Could you check a few things on this model? Use its own coordinates, in mm. Face numbers are marked on the shaded views. Coordinates: 2 decimals unless noted, no trailing zeros. Order: outer loops, then holes, each group sorted by start corner. A loop starts at its lowest first (then second) coordinate and runs counter-clockwise, first axis right, second up. Notation, with made-up numbers: (67.25, 88) -> (94.25, 88) arc R8 ccw to (94.25, 93) -> close; hole circle Ø6 at (3, 27). An arc over 180 degrees is marked (long way). Put each result on its own line as item: value. Start each with the question number.
Q1. If we section it at A-A (x = -5): Please give me the cut outline in (y, z).
Q2. If we section it at B-B (y = -1.25): Please give me the cut outline in (x, z).
Q3. We'd pull the mould along X, two halves only. Please class the marked faces 1, 2, 3 and 4: +X half, -X half, draft (parallel to the pull), parting line (faces both ways), or undercut.
Q4. Will these pins go through, and if not, where does the flat tip stop? pin 1 (1.5 mm diameter, centred on x = -0.5, y = -8.5, fed in from +Z); pin 2 (5 mm diameter, centred on x = -2.5, y = 8, fed in from -Z); pin 3 (2.5 mm diameter, centred on y = 10, z = 2.5, fed in from +X).
Q5. Please list where these lines run through material, in increasing order: line 1 along Y through (x, z) = (-15.2, 2.5); line 2 along Y through (x, z) = (0.5, 7.75); line 3 along Y through (x, z) = (15.35, 2.5).
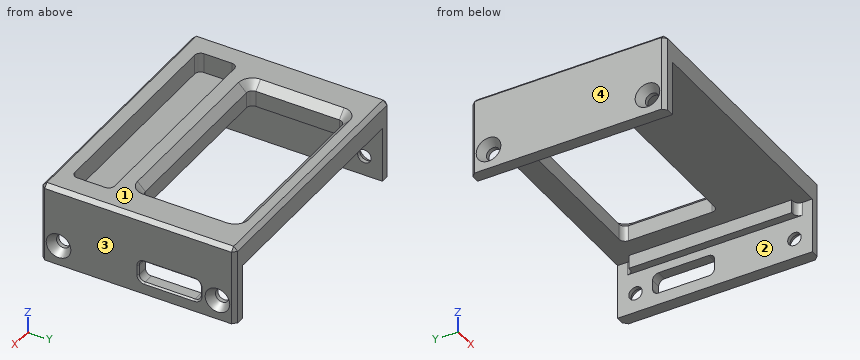
from build123d import *

# Parameters (mm, degrees)
SKETCH1_W           = 32.8
SKETCH1_H           = 24.5
BOSS_EXTRUDE1_DEPTH = 10
SKETCH3_W           = 29.8
SKETCH3_H           = 24.5
CUT_EXTRUDE2_DEPTH  = 5.3
CUT_EXTRUDE3_DEPTH  = 23.782065315
CUT_EXTRUDE4_DEPTH  = 1.5
CHAMFER1_SIZE       = 1
CHAMFER2_SIZE       = 0.2
CHAMFER3_SIZE       = 0.5
CUT_EXTRUDE6_DEPTH  = 2.5
SKETCH10_R          = 0.85
CUT_EXTRUDE7_DEPTH  = 1.5
CUT_EXTRUDE8_START  = -1.5
SKETCH9_R           = 0.85
CUT_EXTRUDE8_DEPTH  = 1.5
CHAMFER7_SIZE       = 0.7
CHAMFER7_SIZE2      = 0.999703605
CHAMFER8_SIZE       = 0.7
CHAMFER8_SIZE2      = 0.999703605
CUT_EXTRUDE11_DEPTH = 1.7


with BuildPart() as part:
    # Sketch1 → Boss-Extrude1 (new body)
    with BuildSketch(Plane.XY):
        Rectangle(SKETCH1_W, SKETCH1_H)
    extrude(amount=BOSS_EXTRUDE1_DEPTH)

    # Sketch3 → Cut-Extrude2 (cut)
    with BuildSketch(Plane(origin=(0, 0, 0), x_dir=(-1, 0, 0), z_dir=(0, 0, -1))):
        Rectangle(SKETCH3_W, SKETCH3_H)
    extrude(amount=-CUT_EXTRUDE2_DEPTH, mode=Mode.SUBTRACT)

    # Sketch4 → Cut-Extrude3 (cut, through all)
    with BuildSketch(Plane.XY.offset(10)):
        with BuildLine():
            Line((-10.75, -2.4), (10.75, -2.4))
            ThreePointArc((10.75, -2.4), (11.280330086, -2.180330086), (11.5, -1.65))
            Line((11.5, -1.65), (11.5, 8.85))
            ThreePointArc((11.5, 8.85), (11.280330086, 9.380330086), (10.75, 9.6))
            Line((10.75, 9.6), (-10.75, 9.6))
            ThreePointArc((-10.75, 9.6), (-11.280330086, 9.380330086), (-11.5, 8.85))
            Line((-11.5, 8.85), (-11.5, -1.65))
            ThreePointArc((-11.5, -1.65), (-11.280330086, -2.180330086), (-10.75, -2.4))
        make_face()
    extrude(amount=-CUT_EXTRUDE3_DEPTH, mode=Mode.SUBTRACT)

    # Sketch5 → Cut-Extrude4 (cut)
    with BuildSketch(Plane(origin=(16.4, 0, 0), x_dir=(0, 0, -1), z_dir=(1, 0, 0))):
        with BuildLine():
            Line((-3.45, 7.85), (-2.25, 7.85))
            ThreePointArc((-2.25, 7.85), (-1.719669914, 7.630330086), (-1.5, 7.1))
            Line((-1.5, 7.1), (-1.5, 0.8))
            ThreePointArc((-1.5, 0.8), (-1.719669914, 0.269669914), (-2.25, 0.05))
            Line((-2.25, 0.05), (-3.45, 0.05))
            ThreePointArc((-3.45, 0.05), (-3.980330086, 0.269669914), (-4.2, 0.8))
            Line((-4.2, 0.8), (-4.2, 7.1))
            ThreePointArc((-4.2, 7.1), (-3.980330086, 7.630330086), (-3.45, 7.85))
        make_face()
    extrude(amount=-CUT_EXTRUDE4_DEPTH, mode=Mode.SUBTRACT)

    # Chamfer1
    chamfer1_edges = [part.edges().sort_by_distance(p)[0] for p in [
        (-11.280330086, -2.180330086, 10),
        (0, -2.4, 10),
        (11.280330086, -2.180330086, 10),
        (11.5, 3.6, 10),
        (11.280330086, 9.380330086, 10),
        (0, 9.6, 10),
        (-11.280330086, 9.380330086, 10),
        (-11.5, 3.6, 10),
    ]]
    chamfer(chamfer1_edges, length=CHAMFER1_SIZE)

    # Chamfer2
    chamfer2_edges = [part.edges().sort_by_distance(p)[0] for p in [
        (16.4, 7.85, 2.85),
        (16.4, 3.95, 1.5),
        (16.4, 7.630330086, 3.980330086),
        (16.4, 3.95, 4.2),
        (16.4, 0.269669914, 3.980330086),
        (16.4, 0.05, 2.85),
        (16.4, 0.269669914, 1.719669914),
        (16.4, 7.630330086, 1.719669914),
    ]]
    chamfer(chamfer2_edges, length=CHAMFER2_SIZE)

    # Chamfer3
    chamfer3_edges = [part.edges().sort_by_distance(p)[0] for p in [
        (-16.4, 0, 10),
        (0, -12.25, 10),
        (16.4, 0, 10),
        (0, 12.25, 10),
        (16.4, -12.25, 5),
        (-16.4, -12.25, 5),
        (-16.4, 12.25, 5),
        (16.4, 12.25, 5),
    ]]
    chamfer(chamfer3_edges, length=CHAMFER3_SIZE)

    # Sketch8 → Cut-Extrude6 (cut)
    with BuildSketch(Plane.XY.offset(10)):
        with BuildLine():
            Line((-12.75, -10.1), (12.75, -10.1))
            ThreePointArc((12.75, -10.1), (13.280330086, -9.880330086), (13.5, -9.35))
            Line((13.5, -9.35), (13.5, -5.85))
            ThreePointArc((13.5, -5.85), (13.280330086, -5.319669914), (12.75, -5.1))
            Line((12.75, -5.1), (-12.75, -5.1))
            ThreePointArc((-12.75, -5.1), (-13.280330086, -5.319669914), (-13.5, -5.85))
            Line((-13.5, -5.85), (-13.5, -9.35))
            ThreePointArc((-13.5, -9.35), (-13.280330086, -9.880330086), (-12.75, -10.1))
        make_face()
    extrude(amount=-CUT_EXTRUDE6_DEPTH, mode=Mode.SUBTRACT)

    # Sketch10 → Cut-Extrude7 (cut)
    with BuildSketch(Plane.ZY.offset(16.4)):
        with Locations((2.5, 10)):
            Circle(SKETCH10_R)
        with Locations((2.5, -10)):
            Circle(SKETCH10_R)
    extrude(amount=-CUT_EXTRUDE7_DEPTH, mode=Mode.SUBTRACT)

    # Sketch9 → Cut-Extrude8 (cut)
    with BuildSketch(Plane(origin=(16.4, 0, 0), x_dir=(0, 0, -1), z_dir=(1, 0, 0)).offset(CUT_EXTRUDE8_START)):
        with Locations(Location((-2.5, -10, 0), (0, 0, 180))):
            Circle(SKETCH9_R)
        with Locations(Location((-2.5, 10, 0), (0, 0, 180))):
            Circle(SKETCH9_R)
    extrude(amount=CUT_EXTRUDE8_DEPTH, mode=Mode.SUBTRACT)

    # Chamfer7
    chamfer7_edges = [part.edges().sort_by_distance(p)[0] for p in [
        (-16.4, 10, 1.65),
        (-16.4, -10, 1.65),
    ]]
    chamfer7_side = [part.faces().sort_by_distance(p)[0] for p in [
        (-16.4, 0, 4.796701497),
    ]]
    chamfer(chamfer7_edges, length=CHAMFER7_SIZE, length2=CHAMFER7_SIZE2, reference=chamfer7_side[0])

    # Chamfer8
    chamfer8_edges = [part.edges().sort_by_distance(p)[0] for p in [
        (16.4, -10, 1.65),
        (16.4, 10, 1.65),
    ]]
    chamfer8_side = [part.faces().sort_by_distance(p)[0] for p in [
        (16.4, -0.501630017, 5.043922739),
    ]]
    chamfer(chamfer8_edges, length=CHAMFER8_SIZE, length2=CHAMFER8_SIZE2, reference=chamfer8_side[0])

    # Sketch15 → Cut-Extrude11 (cut)
    with BuildSketch(Plane(origin=(0, 0, 5.3), x_dir=(-1, 0, 0), z_dir=(0, 0, -1))):
        with BuildLine():
            Line((-14.9, 12.25), (14.9, 12.25))
            Line((14.9, 12.25), (14.9, 11.001705033))
            ThreePointArc((14.9, 11.001705033), (14.680330086, 10.471374947), (14.15, 10.251705033))
            Line((14.15, 10.251705033), (13.900532635, 10.251705033))
            Line((13.900532635, 10.251705033), (13.900532635, -10.246251607))
            Line((13.900532635, -10.246251607), (14.15, -10.246251607))
            ThreePointArc((14.15, -10.246251607), (14.680330086, -10.465921521), (14.9, -10.996251607))
            Line((14.9, -10.996251607), (14.9, -12.25))
            Line((14.9, -12.25), (-14.9, -12.25))
            Line((-14.9, -12.25), (-14.9, -10.996251607))
            ThreePointArc((-14.9, -10.996251607), (-14.680330086, -10.465921521), (-14.15, -10.246251607))
            Line((-14.15, -10.246251607), (-13.902617277, -10.246251607))
            Line((-13.902617277, -10.246251607), (-13.902617277, 10.251705033))
            Line((-13.902617277, 10.251705033), (-14.15, 10.251705033))
            ThreePointArc((-14.15, 10.251705033), (-14.680330086, 10.471374947), (-14.9, 11.001705033))
            Line((-14.9, 11.001705033), (-14.9, 12.25))
        make_face()
    extrude(amount=-CUT_EXTRUDE11_DEPTH, mode=Mode.SUBTRACT)


solid = part.part
The answers:
1. outline: (-12.25, 7) -> (-2.4, 7) -> (-2.4, 9) -> (-3.4, 10) -> (-5.1, 10) -> (-5.1, 7.5) -> (-10.1, 7.5) -> (-10.1, 10) -> (-11.75, 10) -> (-12.25, 9.5) -> close; (9.6, 7) -> (12.25, 7) -> (12.25, 9.5) -> (11.75, 10) -> (10.6, 10) -> (9.6, 9) -> close
2. outline: (-16.4, 0) -> (-14.9, 0) -> (-14.9, 5.3) -> (-13.9, 5.3) -> (-13.9, 7) -> (-11.5, 7) -> (-11.5, 9) -> (-12.5, 10) -> (-15.9, 10) -> (-16.4, 9.5) -> close; (11.5, 7) -> (13.9, 7) -> (13.9, 5.3) -> (14.9, 5.3) -> (14.9, 0) -> (16.4, 0) -> (16.4, 9.5) -> (15.9, 10) -> (12.5, 10) -> (11.5, 9) -> close
3. face 1: draft
3. face 2: undercut
3. face 3: +X half
3. face 4: -X half
4. pin 1: z = 7.5
4. pin 2: z = 7
4. pin 3: x = 15.97
5. line 1: -12.25 to -10.85, -9.15 to 9.15, 10.85 to 12.25
5. line 2: -12.25 to -10.1, -5.1 to -2.4, 9.6 to 12.25
5. line 3: -12.25 to -10.85, -9.15 to 0.05, 7.85 to 9.15, 10.85 to 12.25
